```python
from build123d import *

# Parameters (mm, degrees)
SKETCH1_W           = 50.546
SKETCH1_H           = 42.418
BOSS_EXTRUDE1_DEPTH = 32.258
BOSS_EXTRUDE2_DEPTH = 32.258
SKETCH3_R           = 16.129
BOSS_EXTRUDE3_DEPTH = 90.932
SKETCH5_R           = 16.129
BOSS_EXTRUDE4_DEPTH = 90.932
SKETCH6_R           = 3.937
CUT_EXTRUDE1_DEPTH  = 90.932
SKETCH8_R           = 17.399
BOSS_EXTRUDE5_DEPTH = 11.684
SKETCH9_R           = 7.239
BOSS_EXTRUDE6_DEPTH = 26.67
SKETCH10_W          = 20.32
SKETCH10_H          = 23.876
BOSS_EXTRUDE7_DEPTH = 36.576
SKETCH11_W          = 20.32
SKETCH11_H          = 23.876
BOSS_EXTRUDE8_DEPTH = 36.576
SKETCH12_R          = 4.572
CUT_EXTRUDE2_DEPTH  = 36.576


with BuildPart() as part:
    # Sketch1 → Boss-Extrude1 (new body)
    with BuildSketch(Plane.XY):
        with Locations((25.273, 21.209)):
            Rectangle(SKETCH1_W, SKETCH1_H)
    extrude(amount=BOSS_EXTRUDE1_DEPTH)

    # Sketch2 → Boss-Extrude2 (add)
    with BuildSketch(Plane.XY.offset(32.258)):
        with BuildLine():
            Line((0, 42.418), (11.216038208, 56.368169759))
            ThreePointArc((11.216038208, 56.368169759), (24.775827865, 62.865), (38.335617522, 56.368169759))
            Line((38.335617522, 56.368169759), (50.546, 42.418))
            Line((50.546, 42.418), (0, 42.418))
        make_face()
    extrude(amount=-BOSS_EXTRUDE2_DEPTH)

    # Sketch3 → Boss-Extrude3 (add)
    with BuildSketch(Plane.ZY):
        with Locations((16.129, 24.511)):
            Circle(SKETCH3_R)
    extrude(amount=BOSS_EXTRUDE3_DEPTH)

    # Sketch5 → Boss-Extrude4 (add)
    with BuildSketch(Plane(origin=(50.546, 0, 0), x_dir=(0, 0, -1), z_dir=(1, 0, 0))):
        with Locations((-16.129, 24.511)):
            Circle(SKETCH5_R)
    extrude(amount=BOSS_EXTRUDE4_DEPTH)

    # Sketch6 → Cut-Extrude1 (cut)
    with BuildSketch(Plane.XY.offset(32.258)):
        with Locations((42.291, 7.493)):
            Circle(SKETCH6_R)
        with Locations((8.255, 7.493)):
            Circle(SKETCH6_R)
    extrude(amount=-CUT_EXTRUDE1_DEPTH, mode=Mode.SUBTRACT)

    # Sketch8 → Boss-Extrude5 (add)
    with BuildSketch(Plane.XY.offset(32.258)):
        with Locations((24.775827865, 45.466)):
            Circle(SKETCH8_R)
    extrude(amount=BOSS_EXTRUDE5_DEPTH)

    # Sketch9 → Boss-Extrude6 (add)
    with BuildSketch(Plane.XY.offset(43.942)):
        with Locations((24.775827865, 45.466)):
            Circle(SKETCH9_R)
    extrude(amount=BOSS_EXTRUDE6_DEPTH)

    # Sketch10 → Boss-Extrude7 (add)
    with BuildSketch(Plane(origin=(141.478, 0, 0), x_dir=(0, 0, -1), z_dir=(1, 0, 0))):
        with Locations((-16.129, 24.511)):
            Rectangle(SKETCH10_W, SKETCH10_H)
    extrude(amount=BOSS_EXTRUDE7_DEPTH)

    # Sketch11 → Boss-Extrude8 (add)
    with BuildSketch(Plane.ZY.offset(90.932)):
        with Locations((16.129, 24.511)):
            Rectangle(SKETCH11_W, SKETCH11_H)
    extrude(amount=BOSS_EXTRUDE8_DEPTH)

    # Sketch12 → Cut-Extrude2 (cut)
    with BuildSketch(Plane(origin=(0, 36.449, 0), x_dir=(1, 0, 0), z_dir=(0, 1, 0))):
        with Locations((166.878, -16.129)):
            Circle(SKETCH12_R)
        with Locations((-117.326344271, -16.129)):
            Circle(SKETCH12_R)
    extrude(amount=-CUT_EXTRUDE2_DEPTH, mode=Mode.SUBTRACT)


solid = part.part
```
Could you check a few things on this model? Use its own coordinates, in mm. A direction names the side the tool comes from. Round coordinates to 2 decimals unless told otherwise and drop trailing zeros. Loops run counter-clockwise (first coordinate to the right, second up) from the corner with the lowest first, then second, coordinate; pieces in that order, holes last. Notation, with made-up numbers: M 54.25,50 L 99.25,50 A21 cw 99.25,67 Z; hole C -37,43.25 d2. An arc over 180 degrees is marked long. Put each result on its own line as item: value.
Q1. Imagine slicing it at B-B (z = 54.5). Write out the boundary of the cut face in (x, y), then the cut area to 3 significant figures.
Check result:
outline: C 24.78,45.47 d14.48
area: 165 mm2
Q2. I need wall thicknesses on probe 1 along Y at (x, z) = (25.5, 7); probe 2 along Y at (x, z) = (161, 12); probe 3 along Z at (x, y) = (9, 51). Which ranges of each line are inside material? Lowest first, please.
Check result:
probe 1: 0 to 62.85
probe 2: 12.57 to 36.45
probe 3: 0 to 43.94
Q3. Imagine slicing it at C-C (x = -101.5). Write out the boundary of the cut face in (y, z), then the cut area to 3 significant figures.
Check result:
outline: M 12.57,5.97 L 36.45,5.97 L 36.45,26.29 L 12.57,26.29 Z
area: 485 mm2
Q4. Imagine slicing it at A-A (x = -54.5). Write out the boundary of the cut face in (y, z).
Check result:
outline: C 24.51,16.13 d32.26
Q5. On a 3-axis mill with a long thin cutter (end or side, diameter ignored), from which of +Z, -Z, +X, -X, +Y, -Y can I reach the whole of each face in a straight line? I mean faces 5 (the face through (160, 36.449, 16)), 6 (the face through (31.46, 42.69, 57.09)), 7 (the face through (160, 24, 26.289)), 8 (the face through (-109, 24, 5.969)), 9 (the face through (0, 7, 16)). Say none if no direction works.
Check result:
face 5: +Z, -Z, +X, +Y
face 6: +Z
face 7: +Z, +X, +Y, -Y
face 8: -Z, -X, +Y, -Y
face 9: -X, -Y
Q6. Thinking about a two-plate mould opening in Z: for faces 1 (the face through (26, 32, 0)), 2 (the face through (-112.965, 24.678, 14.756)), 3 (the face through (-109, 12.573, 16)), 4 (the face through (25, 46, 70.612)), which applies, released by +Z, released by -Z, zero draft, split by the parting line, or undercut?
Check result:
face 1: released by -Z
face 2: undercut
face 3: zero draft
face 4: released by +Z
Q7. For pin 1 (14.5 mm diameter, centred on x = -117.33, z = 16.13, fed in from +Y); pin 2 (3 mm diameter, centred on x = -49.5, y = 20, fed in from -Z); pin 3 (12 mm diameter, centred on y = 34, z = 35.5, fed in from +X), each with a flat end and sliding along its axis, tell me the tip position at first contact or that it passes through.
Check result:
pin 1: y = 36.45
pin 2: z = 0.28
pin 3: x = 141.48
